from build123d import *

# Parameters (mm, degrees)
SKETCH1_W           = 130
SKETCH1_H           = 55
BOSS_EXTRUDE1_DEPTH = 2
SKETCH2_W           = 130
SKETCH2_H           = 2
BOSS_EXTRUDE2_DEPTH = 45
SKETCH3_W           = 25
SKETCH3_H           = 55
CUT_EXTRUDE1_DEPTH  = 45
SKETCH4_W           = 3.5
SKETCH4_H           = 11
CUT_EXTRUDE2_DEPTH  = 2
SKETCH6_W           = 80
SKETCH6_H           = 2
BOSS_EXTRUDE3_DEPTH = 55
SKETCH7_R           = 1.75
SKETCH7_R_2         = 5
CUT_EXTRUDE3_DEPTH  = 2
SKETCH8_W           = 80
SKETCH8_H           = 2
BOSS_EXTRUDE4_DEPTH = 30
SKETCH9_W           = 80
SKETCH9_H           = 57
BOSS_EXTRUDE5_DEPTH = 2
SKETCH11_R          = 5
SKETCH11_R_2        = 1.75
SKETCH11_W          = 30.278017406
SKETCH11_H          = 2.009390924
CUT_EXTRUDE4_DEPTH  = 2
SKETCH12_R          = 1.75
CUT_EXTRUDE5_DEPTH  = 2


with BuildPart() as part:
    # Sketch1 → Boss-Extrude1 (new body)
    with BuildSketch(Plane(origin=(0, 0, 0), x_dir=(1, 0, 0), z_dir=(0, 1, 0))):
        Rectangle(SKETCH1_W, SKETCH1_H)
    extrude(amount=BOSS_EXTRUDE1_DEPTH)

    # Sketch2 → Boss-Extrude2 (add)
    with BuildSketch(Plane(origin=(0, 0, 0), x_dir=(1, 0, 0), z_dir=(0, 1, 0))):
        with Locations((0, 28.5)):
            Rectangle(SKETCH2_W, SKETCH2_H)
    extrude(amount=BOSS_EXTRUDE2_DEPTH)

    # Sketch3 → Cut-Extrude1 (cut)
    with BuildSketch(Plane(origin=(0, 2, 0), x_dir=(1, 0, 0), z_dir=(0, 1, 0))):
        with Locations((-52.5, 0)):
            Rectangle(SKETCH3_W, SKETCH3_H)
        with Locations((52.5, 0)):
            Rectangle(SKETCH3_W, SKETCH3_H)
    extrude(amount=-CUT_EXTRUDE1_DEPTH, mode=Mode.SUBTRACT)

    # Sketch4 → Cut-Extrude2 (cut)
    with BuildSketch(Plane.XY.offset(-27.5)):
        with Locations((-63.25, 35.5)):
            Rectangle(SKETCH4_W, SKETCH4_H)
        with Locations((-41.75, 35.5)):
            Rectangle(SKETCH4_W, SKETCH4_H)
        with Locations((41.75, 35.5)):
            Rectangle(SKETCH4_W, SKETCH4_H)
        with Locations((63.25, 35.5)):
            Rectangle(SKETCH4_W, SKETCH4_H)
    extrude(amount=-CUT_EXTRUDE2_DEPTH, mode=Mode.SUBTRACT)

    # Sketch6 → Boss-Extrude3 (add)
    with BuildSketch(Plane.XY.offset(-27.5)):
        with Locations((0, 44)):
            Rectangle(SKETCH6_W, SKETCH6_H)
    extrude(amount=BOSS_EXTRUDE3_DEPTH)

    # Sketch7 → Cut-Extrude3 (cut)
    with BuildSketch(Plane(origin=(0, 45, 0), x_dir=(1, 0, 0), z_dir=(0, 1, 0))):
        with Locations((-35.065858189, 19.292839325)):
            Circle(SKETCH7_R)
        with Locations((15.934141811, -23.707160675)):
            Circle(SKETCH7_R)
        with Locations((32, 19.5)):
            Circle(SKETCH7_R_2)
    extrude(amount=-CUT_EXTRUDE3_DEPTH, mode=Mode.SUBTRACT)

    # Sketch8 → Boss-Extrude4 (add)
    with BuildSketch(Plane(origin=(0, 45, 0), x_dir=(1, 0, 0), z_dir=(0, 1, 0))):
        with Locations((0, 28.5)):
            Rectangle(SKETCH8_W, SKETCH8_H)
    extrude(amount=BOSS_EXTRUDE4_DEPTH)

    # Sketch9 → Boss-Extrude5 (add)
    with BuildSketch(Plane(origin=(0, 75, 0), x_dir=(1, 0, 0), z_dir=(0, 1, 0))):
        with Locations((0, 1)):
            Rectangle(SKETCH9_W, SKETCH9_H)
    extrude(amount=BOSS_EXTRUDE5_DEPTH)

    # Sketch11 → Cut-Extrude4 (cut)
    with BuildSketch(Plane(origin=(0, 77, 0), x_dir=(1, 0, 0), z_dir=(0, 1, 0))):
        with Locations((32, 19.5)):
            Circle(SKETCH11_R)
        with Locations((-7.5, -22.699940475)):
            Circle(SKETCH11_R_2)
        with Locations((7.5, -22.699940475)):
            Circle(SKETCH11_R_2)
        with Locations((0, -18.023076891)):
            Rectangle(SKETCH11_W, SKETCH11_H)
        with Locations((0, 18.023076891)):
            Rectangle(SKETCH11_W, SKETCH11_H)
    extrude(amount=-CUT_EXTRUDE4_DEPTH, mode=Mode.SUBTRACT)

    # Sketch12 → Cut-Extrude5 (cut)
    with BuildSketch(Plane.XZ):
        with Locations((-16.693132279, 20.191612333)):
            Circle(SKETCH12_R)
        with Locations((16.693132279, -20.97095973)):
            Circle(SKETCH12_R)
    extrude(amount=-CUT_EXTRUDE5_DEPTH, mode=Mode.SUBTRACT)


solid = part.part
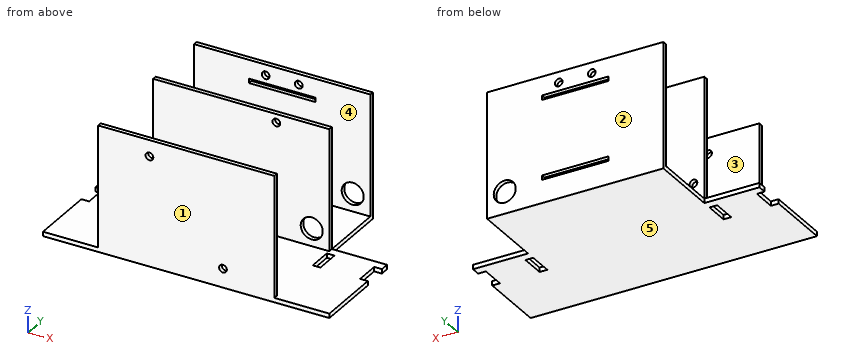
Build history of the part. All positions in model axes, mm. Face numbers are marked on the shaded views. A direction names the side the tool comes from. Round coordinates to 2 decimals unless told otherwise and drop trailing zeros. Write each loop counter-clockwise with the first axis right and the second up, starting at its lowest first coordinate (ties: lowest second). Pieces come first, ordered by that corner, then holes. Notation, with made-up numbers: (8.25, 89) - (27.25, 89) arc R12 cw to (27.25, 111) - close; hole circle Ø8 at (-6, 9.5). An arc over 180 degrees is marked (long way). One line per question, with ' | ' between items.
1. Drill centre lines: line 1 along Y through (x, z) = (23, -26.5); line 2 along X through (y, z) = (76.55, -19.5); line 3 along Z through (x, y) = (49, 29.5). Where is each one in solid material? Low to high. Write a range as from..to.
Results are:
line 1: 0..2, 43..45, 75..77 | line 2: -40..27, 37..40 | line 3: -29.5..-27.5
2. Drop flat-ended pins along their axis: pin 1 Ø0.6 at (y, z) = (43.5, -12.5) entering from +X; pin 2 Ø1 at (y, z) = (37.5, -28) entering from +X; pin 3 Ø2 at (x, z) = (57, -28) entering from +Y. Give the stop position or say it passes through.
Results are:
pin 1: x = 40 | pin 2: x = 61.5 | pin 3: y = 45
3. Band-saw the part on D-D, the plane x = 32. Write the cut outline in (y, z).
Results are:
outline: (0, -29.5) - (77, -29.5) - (77, -24.5) - (75, -24.5) - (75, -27.5) - (45, -27.5) - (45, -24.5) - (43, -24.5) - (43, -27.5) - (2, -27.5) - (2, 27.5) - (0, 27.5) - close; (43, -14.5) - (45, -14.5) - (45, 27.5) - (43, 27.5) - close; (75, -14.5) - (77, -14.5) - (77, 27.5) - (75, 27.5) - close
4. Tool access for the marked faces 4 and 5: list every direction of +Z, -Z, +X, -X, +Y, -Y with a clear straight run to the whole face (end or side of a thin tool).
Results are:
face 4: +Z, +X, -X | face 5: -Z, +X, -X, +Y, -Y
5. Mould opens along Y. For the marked faces 1, 2 and 3 say: released by +Y, released by -Y, zero draft, split by the parting line, or undercut.
Results are:
face 1: released by -Y | face 2: released by +Y | face 3: undercut
6. Band-saw the part on B-B, the plane x = -7.5. Write the cut outline in (y, z).
Results are:
outline: (0, -29.5) - (77, -29.5) - (77, -19.03) - (75, -19.03) - (75, -27.5) - (45, -27.5) - (45, 27.5) - (43, 27.5) - (43, -27.5) - (2, -27.5) - (2, 27.5) - (0, 27.5) - close; (75, -17.02) - (77, -17.02) - (77, 17.02) - (75, 17.02) - close; (75, 19.03) - (77, 19.03) - (77, 20.95) - (75, 20.95) - close; (75, 24.45) - (77, 24.45) - (77, 27.5) - (75, 27.5) - close
7. Band-saw the part on C-C, the plane z = -9.5. Write the cut outline in (x, y), and give its area (3 significant figures).
Results are:
outline: (-40, 0) - (40, 0) - (40, 2) - (-40, 2) - close; (-40, 43) - (40, 43) - (40, 45) - (-40, 45) - close; (-40, 75) - (40, 75) - (40, 77) - (-40, 77) - close | area: 480 mm^2
8. Band-saw the part on A-A, the plane y = 32. Write the cut outline in (x, z).
Results are:
outline: (-61.5, -29.5) - (-43.5, -29.5) - (-43.5, -27.5) - (-61.5, -27.5) - close; (-40, -29.5) - (40, -29.5) - (40, -27.5) - (-40, -27.5) - close; (43.5, -29.5) - (61.5, -29.5) - (61.5, -27.5) - (43.5, -27.5) - close
